from build123d import *

# Parameters (mm, degrees)
SKETCH1_W           = 152.4
SKETCH1_H           = 101.6
BOSS_EXTRUDE1_DEPTH = 135
SKETCH2_W           = 104
SKETCH2_H           = 78
CUT_EXTRUDE1_DEPTH  = 6
SKETCH4_R           = 7
BOSS_EXTRUDE3_DEPTH = 60
SKETCH5_R           = 4.5
CUT_EXTRUDE3_DEPTH  = 80
SKETCH12_W          = 100
SKETCH12_H          = 75.5
CUT_EXTRUDE7_DEPTH  = 120
SKETCH13_W          = 60
SKETCH13_H          = 42
CUT_EXTRUDE8_DEPTH  = 2
SKETCH24_R          = 2.5
CUT_EXTRUDE9_DEPTH  = 15
SKETCH26_W          = 10
SKETCH26_H          = 20
CUT_EXTRUDE10_DEPTH = 27.2


with BuildPart() as part:
    # Sketch1 → Boss-Extrude1 (new body)
    with BuildSketch(Plane.XY):
        Rectangle(SKETCH1_W, SKETCH1_H)
    extrude(amount=BOSS_EXTRUDE1_DEPTH)

    # Sketch2 → Cut-Extrude1 (cut)
    with BuildSketch(Plane(origin=(0, 0, 0), x_dir=(-1, 0, 0), z_dir=(0, 0, -1))):
        Rectangle(SKETCH2_W, SKETCH2_H)
    extrude(amount=-CUT_EXTRUDE1_DEPTH, mode=Mode.SUBTRACT)

    # Sketch4 → Boss-Extrude3 (add)
    with BuildSketch(Plane(origin=(0, 0, 0), x_dir=(-1, 0, 0), z_dir=(0, 0, -1))):
        with Locations((-64.1, -30.8)):
            Circle(SKETCH4_R)
        with Locations((-64.1, 30.8)):
            Circle(SKETCH4_R)
        with Locations((64.1, 30.8)):
            Circle(SKETCH4_R)
        with Locations((64.1, -30.8)):
            Circle(SKETCH4_R)
    extrude(amount=BOSS_EXTRUDE3_DEPTH)

    # Sketch5 → Cut-Extrude3 (cut)
    with BuildSketch(Plane(origin=(0, 0, -60), x_dir=(-1, 0, 0), z_dir=(0, 0, -1))):
        with Locations((-64.1, 30.8)):
            Circle(SKETCH5_R)
        with Locations((64.1, 30.8)):
            Circle(SKETCH5_R)
        with Locations((64.1, -30.8)):
            Circle(SKETCH5_R)
        with Locations((-64.1, -30.8)):
            Circle(SKETCH5_R)
    extrude(amount=-CUT_EXTRUDE3_DEPTH, mode=Mode.SUBTRACT)

    # Sketch12 → Cut-Extrude7 (cut)
    with BuildSketch(Plane(origin=(0, 0, 6), x_dir=(-1, 0, 0), z_dir=(0, 0, -1))):
        Rectangle(SKETCH12_W, SKETCH12_H)
    extrude(amount=-CUT_EXTRUDE7_DEPTH, mode=Mode.SUBTRACT)

    # Sketch13 → Cut-Extrude8 (cut)
    with BuildSketch(Plane(origin=(0, 0, 126), x_dir=(-1, 0, 0), z_dir=(0, 0, -1))):
        with Locations((0, 4.75)):
            Rectangle(SKETCH13_W, SKETCH13_H)
    extrude(amount=-CUT_EXTRUDE8_DEPTH, mode=Mode.SUBTRACT)

    # Sketch24 → Cut-Extrude9 (cut)
    with BuildSketch(Plane.ZY.offset(-50)):
        with Locations((12.5, 30.8)):
            Circle(SKETCH24_R)
        with Locations((12.5, -30.8)):
            Circle(SKETCH24_R)
    cut_extrude9 = extrude(amount=-CUT_EXTRUDE9_DEPTH, mode=Mode.SUBTRACT)

    # Mirror2: Cut-Extrude9 across plane
    add(cut_extrude9.mirror(Plane(origin=(0, 0, 0), x_dir=(0, 0, 1), z_dir=(1, 0, 0))), mode=Mode.SUBTRACT)

    # Sketch26 → Cut-Extrude10 (cut, through all)
    with BuildSketch(Plane.ZY.offset(-50)):
        with Locations((115, -25.8)):
            Rectangle(SKETCH26_W, SKETCH26_H)
    extrude(amount=-CUT_EXTRUDE10_DEPTH, mode=Mode.SUBTRACT)


solid = part.part
The listing builds one solid part. Answer for the finished solid, in the listing's coordinates (mm). A direction names the side the tool comes from. Round coordinates to 2 decimals unless told otherwise and drop trailing zeros. Order: outer loops, then holes, each group sorted by start corner. A loop starts at its lowest first (then second) coordinate and runs counter-clockwise, first axis right, second up. Notation, with made-up numbers: (-24, -12.5) -> (-2, -12.5) arc R20 ccw to (-2, 14.5) -> close; hole circle Ø5 at (-19.5, 32.5). An arc over 180 degrees is marked (long way). Put each result on its own line as item: value.
Q1. Each of these flat-tipped pins is pushed along its axis until it touches: P1, Ø8, axis at x = 21, y = 39, coming from the -Z side; P2, Ø5.5, axis at x = -64.1, y = 30.8, coming from the -Z side; P3, Ø1.5, axis at x = 60.5, z = -3.5, coming from the -Y side; P4, Ø6, axis at x = 52.5, z = -29.5, coming from the +Y side. Where does it stop, or does it pass through?
Results list:
P1: z = 0
P2: z = 20
P3: y = -37.19
P4: through
Q2. Determine the mould class of faces 4 (the flat face through (1, -25, 126)), 5 (the cylindrical face through (57.423, 32.903, -29.58)), 6 (the flat face through (63, -26, 110)) for opening direction Z: pulls with the +Z half, pulls with the -Z half, needs draft (parallel to the pull), parting line crosses it, or undercut.
Results list:
face 4: pulls with the -Z half
face 5: needs draft
face 6: undercut
Q3. Which of the six approach directions +Z, -Z, +X, -X, +Y, -Y give full straight-line access (tool end or side, diameter ignored) to faces 1 (the flat face through (1, -39, 3)), 2 (the flat face through (63, -35.8, 115)), 3 (the cylindrical face through (55.1, -30.7, 10))?
Results list:
face 1: -Z
face 2: +X
face 3: none
Q4. Section A-A, the plane z = 12.5 is taken. Write down the section's boundary in (x, y), and give its area (3 significant figures).
Results list:
outline: (-76.2, -50.8) -> (76.2, -50.8) -> (76.2, 50.8) -> (-76.2, 50.8) -> close; hole (-60.36, -33.3) -> (-50, -33.3) -> (-50, -37.75) -> (50, -37.75) -> (50, -33.3) -> (60.36, -33.3) arc R4.5 ccw (long way) to (60.36, -28.3) -> (50, -28.3) -> (50, 28.3) -> (60.36, 28.3) arc R4.5 ccw (long way) to (60.36, 33.3) -> (50, 33.3) -> (50, 37.75) -> (-50, 37.75) -> (-50, 33.3) -> (-60.36, 33.3) arc R4.5 ccw (long way) to (-60.36, 28.3) -> (-50, 28.3) -> (-50, -28.3) -> (-60.36, -28.3) arc R4.5 ccw (long way) to start
area: 7,480 mm^2
Q5. Consider line 1 along Y through (x, z) = (-54.25, 12.5); line 2 along Y through (x, z) = (64.1, -10); line 3 along Y through (x, z) = (34, 24.5). Determine where each line is inside the solid, lowest interval first.
Results list:
line 1: -50.8 to -33.3, -28.3 to 28.3, 33.3 to 50.8
line 2: -37.8 to -35.3, -26.3 to -23.8, 23.8 to 26.3, 35.3 to 37.8
line 3: -50.8 to -37.75, 37.75 to 50.8
Q6. Section C-C, the plane y = 30.8 is taken. Count the separate pieces of the cut face and the enclosed holes in it, and give its area (3 significant figures).
Results list:
separate pieces: 3
enclosed holes: 0
area: 8,090 mm^2
Q7. Section B-B, the plane x = 64.1 is taken. Write down the section's boundary in (y, z), and give its area (3 significant figures).
Results list:
outline: (-50.8, 0) -> (-37.8, 0) -> (-37.8, -60) -> (-35.3, -60) -> (-35.3, 20) -> (-26.3, 20) -> (-26.3, -60) -> (-23.8, -60) -> (-23.8, 0) -> (23.8, 0) -> (23.8, -60) -> (26.3, -60) -> (26.3, 20) -> (35.3, 20) -> (35.3, -60) -> (37.8, -60) -> (37.8, 0) -> (50.8, 0) -> (50.8, 135) -> (-50.8, 135) -> close; hole (-35.8, 110) -> (-15.8, 110) -> (-15.8, 120) -> (-35.8, 120) -> close
area: 13,800 mm^2
